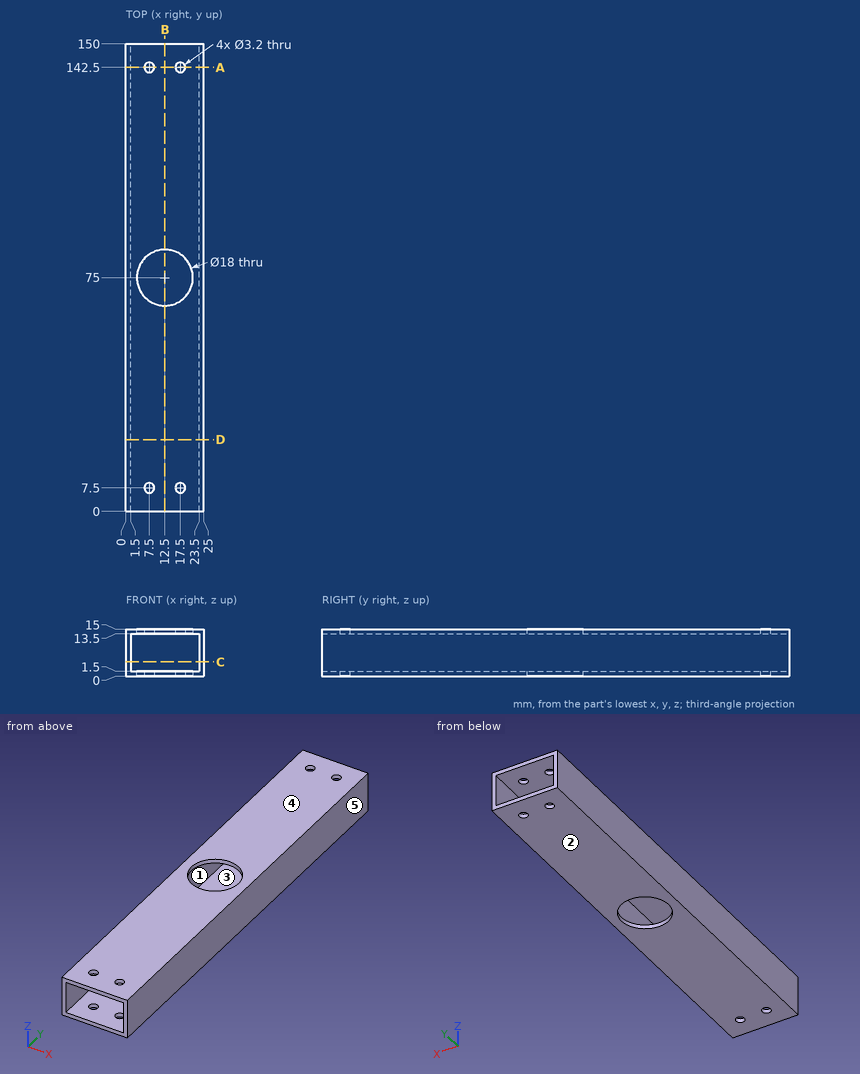
Print and shaded views of the part. All mm, measured from the part's lowest x, y and z. A direction names the side the tool comes from. Coordinates: 2 decimals unless noted, no trailing zeros. Write each loop counter-clockwise with the first axis right and the second up, starting at its lowest first coordinate (ties: lowest second). Pieces come first, ordered by that corner, then holes. Notation, with made-up numbers: M 24,-10.75 L 81,-10.75 A14 cw 81,-4.75 Z; hole C 80,-23.5 d1. An arc over 180 degrees is marked long. Return JSON: item names as keys, results as strings.
1. Saw through at C-C, the plane z = 4.5. Write the cut outline in (x, y), then the cut area to 3 significant figures.
Determined:
{"outline": "M 0,0 L 1.5,0 L 1.5,150 L 0,150 Z; M 23.5,0 L 25,0 L 25,150 L 23.5,150 Z", "area": "450 mm²"}
2. Probe L1, parallel to X at y = 142.5, z = 14.5; L2, parallel to Z at x = 4.5, y = 130.5; L3, parallel to X at y = 34.5, z = 2. List the from-to ranges inside material, lowest first.
Determined:
{"L1": "0 to 5.9, 9.1 to 15.9, 19.1 to 25", "L2": "0 to 1.5, 13.5 to 15", "L3": "0 to 1.5, 23.5 to 25"}
3. Saw through at D-D, the plane y = 23. Write the cut outline in (x, z), then the cut area to 3 significant figures.
Determined:
{"outline": "M 0,0 L 25,0 L 25,15 L 0,15 Z; hole M 1.5,1.5 L 23.5,1.5 L 23.5,13.5 L 1.5,13.5 Z", "area": "111 mm²"}
4. 3-axis set-ups, long thin cutter, end or side, ignore diameter. For the marked faces 1 and 2: which of +Z, -Z, +X, -X, +Y, -Y reach the whole face in a straight line?
Determined:
{"face 1": "+Y, -Y", "face 2": "-Z, +X, -X, +Y, -Y"}
5. Pull direction Z, two halves, no side cores. Call the marked faces 3, 4 and 5: pulls with the +Z half, pulls with the -Z half, needs draft (parallel to the pull), parting line crosses it, or undercut.
Determined:
{"face 3": "undercut", "face 4": "pulls with the +Z half", "face 5": "needs draft"}
6. Saw through at A-A, the plane y = 142.5. Write the cut outline in (x, z).
Determined:
{"outline": "M 0,0 L 5.9,0 L 5.9,1.5 L 1.5,1.5 L 1.5,13.5 L 5.9,13.5 L 5.9,15 L 0,15 Z; M 9.1,0 L 15.9,0 L 15.9,1.5 L 9.1,1.5 Z; M 9.1,13.5 L 15.9,13.5 L 15.9,15 L 9.1,15 Z; M 19.1,0 L 25,0 L 25,15 L 19.1,15 L 19.1,13.5 L 23.5,13.5 L 23.5,1.5 L 19.1,1.5 Z"}
7. Saw through at B-B, the plane x = 12.5. Write the cut outline in (y, z).
Determined:
{"outline": "M 0,0 L 66,0 L 66,1.5 L 0,1.5 Z; M 0,13.5 L 66,13.5 L 66,15 L 0,15 Z; M 84,0 L 150,0 L 150,1.5 L 84,1.5 Z; M 84,13.5 L 150,13.5 L 150,15 L 84,15 Z"}
